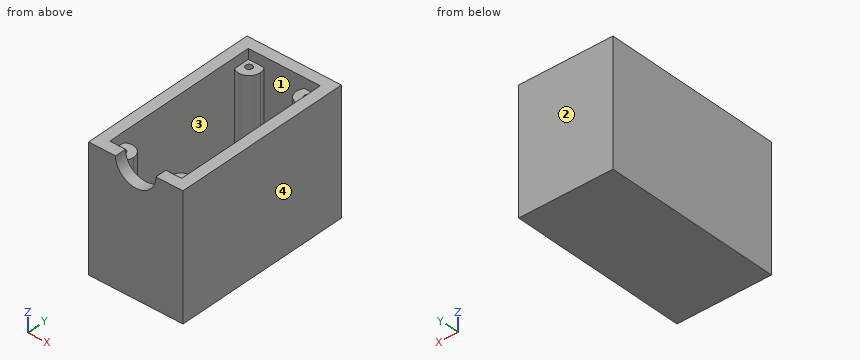
from build123d import *

# Parameters (mm, degrees)
F0_W     = 21
F0_H     = 40
F1_DEPTH = 25
F0_R     = 0.75
F2_DEPTH = 22.75
F3_W     = 21
F3_H     = 40
F4_DEPTH = 2.5
F5_R     = 4.5
F6_DEPTH = 2.5


# Not quite as in the source:
# - a feature names something its author has since deleted; it is built from what else it names


with BuildPart() as f1:
    # F0 (on Top) → F1 (new body)
    with BuildSketch(Plane.XY):
        Rectangle(F0_W, F0_H)
        with BuildLine():
            ThreePointArc((-8, 13.996502206), (-8.2693131131, 17.7627216453), (-4.5026281309, 17.5))
            Line((-4.5026281309, 17.5), (4.5026281309, 17.5))
            ThreePointArc((4.5026281309, 17.5), (7.2926444119, 18.3675177766), (9, 15.996502206))
            ThreePointArc((9, 15.996502206), (8.7360679775, 14.8784682172), (8, 13.996502206))
            Line((8, 13.996502206), (8, -13.9965024172))
            ThreePointArc((8, -13.9965024172), (8.7360679775, -14.8784684285), (9, -15.9965024172))
            ThreePointArc((9, -15.9965024172), (7.2926442865, -18.3675180298), (4.5026279719, -17.5))
            Line((4.5026279719, -17.5), (-4.4973814273, -17.5))
            ThreePointArc((-4.4973814273, -17.5), (-8.2662214687, -17.7728088813), (-8, -14.003497794))
            Line((-8, -14.003497794), (-8, 13.996502206))
        make_face(mode=Mode.SUBTRACT)
        with BuildLine():
            Line((-8, -17.5), (-8, -14.003497794))
            ThreePointArc((-8, -14.003497794), (-8.2662214687, -17.7728088813), (-4.4973814273, -17.5))
            Line((-4.4973814273, -17.5), (-8, -17.5))
        make_face()
        with BuildLine():
            Line((-8, 13.996502206), (-8, 17.5))
            Line((-8, 17.5), (-4.5026281309, 17.5))
            ThreePointArc((-4.5026281309, 17.5), (-8.2693131131, 17.7627216453), (-8, 13.996502206))
        make_face()
        with BuildLine():
            ThreePointArc((9, 15.996502206), (7.2926444119, 18.3675177766), (4.5026281309, 17.5))
            Line((4.5026281309, 17.5), (8, 17.5))
            Line((8, 17.5), (8, 13.996502206))
            ThreePointArc((8, 13.996502206), (8.7360679775, 14.8784682172), (9, 15.996502206))
        make_face()
        with BuildLine():
            ThreePointArc((9, -15.9965024172), (8.7360679775, -14.8784684285), (8, -13.9965024172))
            Line((8, -13.9965024172), (8, -17.5))
            Line((8, -17.5), (4.5026279719, -17.5))
            ThreePointArc((4.5026279719, -17.5), (7.2926442865, -18.3675180298), (9, -15.9965024172))
        make_face()
    extrude(amount=F1_DEPTH)

    # F0 (on Top) → F2 (join)
    with BuildSketch(Plane.XY):
        with BuildLine():
            Line((-4.5026281309, 17.5), (-8, 17.5))
            Line((-8, 17.5), (-8, 13.996502206))
            ThreePointArc((-8, 13.996502206), (-5.3819660113, 13.7604342285), (-4, 15.996502206))
            ThreePointArc((-4, 15.996502206), (-4.1289844293, 16.7891466178), (-4.5026281309, 17.5))
        make_face()
        with Locations((-6.5, 15.996502206)):
            Circle(F0_R, mode=Mode.SUBTRACT)
        with BuildLine():
            Line((8, 17.5), (4.5026281309, 17.5))
            ThreePointArc((4.5026281309, 17.5), (4.7306868869, 14.2302827667), (8, 13.996502206))
            Line((8, 13.996502206), (8, 17.5))
        make_face()
        with Locations((6.5, 15.996502206)):
            Circle(F0_R, mode=Mode.SUBTRACT)
        with BuildLine():
            Line((8, -17.5), (8, -13.9965024172))
            ThreePointArc((8, -13.9965024172), (4.7306869803, -14.2302828844), (4.5026279719, -17.5))
            Line((4.5026279719, -17.5), (8, -17.5))
        make_face()
        with Locations((6.5, -15.9965024172)):
            Circle(F0_R, mode=Mode.SUBTRACT)
        with BuildLine():
            ThreePointArc((-4, -16.003497794), (-5.3819660113, -13.7674298165), (-8, -14.003497794))
            Line((-8, -14.003497794), (-8, -17.5))
            Line((-8, -17.5), (-4.4973814273, -17.5))
            ThreePointArc((-4.4973814273, -17.5), (-4.1276018007, -16.7919943281), (-4, -16.003497794))
        make_face()
        with Locations((-6.5, -16.003497794)):
            Circle(F0_R, mode=Mode.SUBTRACT)
    extrude(amount=F2_DEPTH)

    # F3 (on face) → F4 (join)
    with BuildSketch(Plane.XY):
        Rectangle(F3_W, F3_H)
    extrude(amount=-F4_DEPTH)

    # F5 (on face) → F6 (cut)
    with BuildSketch(Plane.XZ.offset(20)):
        with Locations((0, 25)):
            Circle(F5_R)
    extrude(amount=-F6_DEPTH, mode=Mode.SUBTRACT)


solid = f1.part
Can you work these out from the model? Positions are in its coordinate system, mm. Face numbers are marked on the shaded views. Coordinates: 2 decimals unless noted, no trailing zeros. Loops run counter-clockwise (first coordinate to the right, second up) from the corner with the lowest first, then second, coordinate; pieces in that order, holes last. Notation, with made-up numbers: (82, 64) - (97, 64) arc R29 cw to (97, 92) - close; hole circle Ø1 at (7.25, 84). An arc over 180 degrees is marked (long way). Put each result on its own line as item: value. Start each with the question number.
Item 1: For pin 1 (1.2 mm diameter, centred on x = -6.5, y = -14.5, fed in from +Z), with a flat end and sliding along its axis, tell me the tip position at first contact or that it passes through.
Item 2: Suppose I cut it at B-B (z = 6.5). Please give me the cut outline in (x, y), and give its area (3 significant figures).
Item 3: Suppose I cut it at C-C (y = -8.5). Please give me the cut outline in (x, z), and give its area (4 significant figures).
Item 4: Suppose I cut it at D-D (x = 6.5). Please give me the cut outline in (y, z), and give its area (3 significant figures).
Item 5: If we mould it in two halves opening along Y, with no side actions, what happens to the marked faces 1, 2, 3 and 4? For each: +Y half, -Y half, draft (parallel to the pull), parting line (faces both ways), or undercut.
Item 6: Suppose I cut it at A-A (x = 0). Please give me the cut outline in (y, z).
Item 7: If I drill on line 1 along X through (y, z) = (-16, 22.5); line 2 along Y through (x, z) = (6.5, 5.75); line 3 along X through (y, z) = (-7, 20.25), over which ranges is the centre line in solid material (lowest first)?
Here are the results:
1. pin 1: z = 22.75
2. outline: (-10.5, -20) - (10.5, -20) - (10.5, 20) - (-10.5, 20) - close; hole (-8, -14) arc R2.5 cw to (-4.5, -17.5) - (4.5, -17.5) arc R2.5 cw to (8, -14) - (8, 14) arc R2.5 cw to (4.5, 17.5) - (-4.5, 17.5) arc R2.5 cw to (-8, 14) - close; hole circle Ø1.5 at (-6.5, -16); hole circle Ø1.5 at (-6.5, 16); hole circle Ø1.5 at (6.5, -16); hole circle Ø1.5 at (6.5, 16)
2. area: 330 mm²
3. outline: (-10.5, -2.5) - (10.5, -2.5) - (10.5, 25) - (8, 25) - (8, 0) - (-8, 0) - (-8, 25) - (-10.5, 25) - close
3. area: 177.5 mm²
4. outline: (-20, -2.5) - (20, -2.5) - (20, 25) - (17.5, 25) - (17.5, 22.75) - (16.75, 22.75) - (16.75, 0) - (15.25, 0) - (15.25, 22.75) - (13.5, 22.75) - (13.5, 0) - (-13.5, 0) - (-13.5, 22.75) - (-15.25, 22.75) - (-15.25, 0) - (-16.75, 0) - (-16.75, 22.75) - (-17.5, 22.75) - (-17.5, 25) - (-20, 25) - close
4. area: 339 mm²
5. face 1: undercut
5. face 2: +Y half
5. face 3: undercut
5. face 4: draft
6. outline: (-20, -2.5) - (20, -2.5) - (20, 25) - (17.5, 25) - (17.5, 0) - (-17.5, 0) - (-17.5, 20.5) - (-20, 20.5) - close
7. line 1: -10.5 to -7.25, -5.75 to -4, 4 to 5.75, 7.25 to 10.5
7. line 2: -20 to -16.75, -15.25 to -13.5, 13.5 to 15.25, 16.75 to 20
7. line 3: -10.5 to -8, 8 to 10.5
